```python
from build123d import *

# Parameters (mm, degrees)
SKETCH1_R           = 3.3274
BOSS_EXTRUDE1_DEPTH = 19.05


with BuildPart() as part:
    # Sketch1 → Boss-Extrude1 (new body, symmetric)
    with BuildSketch(Plane.XY):
        with BuildLine():
            Line((-4.064, 16.539617552), (-4.064, 17.496382454))
            ThreePointArc((-4.064, 17.496382454), (-4.519044044, 18.594955958), (-5.617617547, 19.050000004))
            Line((-5.617617547, 19.050000004), (-15.84748704, 19.050000004))
            ThreePointArc((-15.84748704, 19.050000004), (-18.12017629, 18.120192086), (-19.050000001, 15.847509297))
            Line((-19.050000001, 15.847509297), (-19.050000001, 5.617617549))
            ThreePointArc((-19.050000001, 5.617617549), (-18.594955957, 4.519044045), (-17.496382454, 4.064))
            Line((-17.496382454, 4.064), (-16.539617549, 4.064))
            ThreePointArc((-16.539617549, 4.064), (-15.441044044, 4.519044045), (-14.986, 5.617617549))
            Line((-14.986, 5.617617549), (-14.986, 9.385342517))
            ThreePointArc((-14.986, 9.385342517), (-14.721898184, 10.022940701), (-14.0843, 10.287042517))
            Line((-14.0843, 10.287042517), (-13.516042086, 10.287042517))
            ThreePointArc((-13.516042086, 10.287042517), (-13.170975923, 10.218404479), (-12.878443117, 10.022939917))
            Line((-12.878443117, 10.022939917), (-8.14758008, 5.292065242))
            ThreePointArc((-8.14758008, 5.292065242), (-7.117955877, 3.751120652), (-6.756399998, 1.933453582))
            Line((-6.756399998, 1.933453582), (-6.756399998, -1.933453584))
            ThreePointArc((-6.756399998, -1.933453584), (-7.117955877, -3.751120652), (-8.147580078, -5.292065242))
            Line((-8.147580078, -5.292065242), (-12.878443116, -10.022939917))
            ThreePointArc((-12.878443116, -10.022939917), (-13.170975922, -10.21840448), (-13.516042086, -10.287042518))
            Line((-13.516042086, -10.287042518), (-14.0843, -10.287042518))
            ThreePointArc((-14.0843, -10.287042518), (-14.721898185, -10.022940703), (-14.986, -9.385342518))
            Line((-14.986, -9.385342518), (-14.986, -5.617617549))
            ThreePointArc((-14.986, -5.617617549), (-15.441044044, -4.519044046), (-16.539617547, -4.064))
            Line((-16.539617547, -4.064), (-17.496382452, -4.064))
            ThreePointArc((-17.496382452, -4.064), (-18.594955956, -4.519044044), (-19.050000001, -5.617617547))
            Line((-19.050000001, -5.617617547), (-19.050000001, -15.84751072))
            ThreePointArc((-19.050000001, -15.84751072), (-18.120175718, -18.120192644), (-15.84748687, -19.050000001))
            Line((-15.84748687, -19.050000001), (-5.617617549, -19.050000001))
            ThreePointArc((-5.617617549, -19.050000001), (-4.519044046, -18.594955957), (-4.064, -17.496382454))
            Line((-4.064, -17.496382454), (-4.064, -16.539617549))
            ThreePointArc((-4.064, -16.539617549), (-4.519044045, -15.441044044), (-5.617617549, -14.985999999))
            Line((-5.617617549, -14.985999999), (-9.3853, -14.985999999))
            ThreePointArc((-9.3853, -14.985999999), (-10.022898185, -14.721898184), (-10.287, -14.084299999))
            Line((-10.287, -14.084299999), (-10.287, -13.552357131))
            ThreePointArc((-10.287, -13.552357131), (-10.218362387, -13.207291993), (-10.022898969, -12.914759731))
            Line((-10.022898969, -12.914759731), (-5.252158104, -8.14400713))
            ThreePointArc((-5.252158104, -8.14400713), (-3.715177371, -7.117027388), (-1.902183976, -6.7564))
            Line((-1.902183976, -6.7564), (1.902183976, -6.7564))
            ThreePointArc((1.902183976, -6.7564), (3.715177372, -7.117027388), (5.252158106, -8.144007132))
            Line((5.252158106, -8.144007132), (10.022898969, -12.91475973))
            ThreePointArc((10.022898969, -12.91475973), (10.218362387, -13.207291993), (10.287000001, -13.552357132))
            Line((10.287000001, -13.552357132), (10.287000001, -14.0843))
            ThreePointArc((10.287000001, -14.0843), (10.022898185, -14.721898184), (9.385300001, -14.986))
            Line((9.385300001, -14.986), (5.617617549, -14.986))
            ThreePointArc((5.617617549, -14.986), (4.519044045, -15.441044044), (4.064, -16.539617547))
            Line((4.064, -16.539617547), (4.064, -17.496382452))
            ThreePointArc((4.064, -17.496382452), (4.519044043, -18.594955955), (5.617617546, -19.050000001))
            Line((5.617617546, -19.050000001), (15.847486867, -19.050000001))
            ThreePointArc((15.847486867, -19.050000001), (18.120175716, -18.120192646), (19.05, -15.847510723))
            Line((19.05, -15.847510723), (19.05, -5.617617549))
            ThreePointArc((19.05, -5.617617549), (18.594955955, -4.519044045), (17.496382451, -4.064))
            Line((17.496382451, -4.064), (16.539617548, -4.064))
            ThreePointArc((16.539617548, -4.064), (15.441044044, -4.519044045), (14.985999999, -5.617617549))
            Line((14.985999999, -5.617617549), (14.985999999, -9.385342517))
            ThreePointArc((14.985999999, -9.385342517), (14.721898184, -10.022940701), (14.084299999, -10.287042517))
            Line((14.084299999, -10.287042517), (13.516042085, -10.287042517))
            ThreePointArc((13.516042085, -10.287042517), (13.170975922, -10.218404479), (12.878443117, -10.022939917))
            Line((12.878443117, -10.022939917), (8.147580079, -5.292065242))
            ThreePointArc((8.147580079, -5.292065242), (7.117955877, -3.751120652), (6.756399998, -1.933453583))
            Line((6.756399998, -1.933453583), (6.756399998, 1.933453583))
            ThreePointArc((6.756399998, 1.933453583), (7.117955877, 3.751120652), (8.147580078, 5.292065242))
            Line((8.147580078, 5.292065242), (12.878443116, 10.022939916))
            ThreePointArc((12.878443116, 10.022939916), (13.170975922, 10.218404477), (13.516042084, 10.287042515))
            Line((13.516042084, 10.287042515), (14.084299998, 10.287042515))
            ThreePointArc((14.084299998, 10.287042515), (14.721898183, 10.0229407), (14.985999998, 9.385342515))
            Line((14.985999998, 9.385342515), (14.985999998, 5.617617546))
            ThreePointArc((14.985999998, 5.617617546), (15.441044043, 4.519044042), (16.539617547, 4.063999997))
            Line((16.539617547, 4.063999997), (17.49638245, 4.063999997))
            ThreePointArc((17.49638245, 4.063999997), (18.594955956, 4.519044042), (19.05, 5.617617548))
            Line((19.05, 5.617617548), (19.05, 15.8475093))
            ThreePointArc((19.05, 15.8475093), (18.120176289, 18.120192086), (15.847487041, 19.050000004))
            Line((15.847487041, 19.050000004), (5.617617548, 19.050000004))
            ThreePointArc((5.617617548, 19.050000004), (4.519044044, 18.594955959), (4.063999999, 17.496382454))
            Line((4.063999999, 17.496382454), (4.063999999, 16.539617552))
            ThreePointArc((4.063999999, 16.539617552), (4.519044044, 15.441044047), (5.617617548, 14.986000002))
            Line((5.617617548, 14.986000002), (9.385299999, 14.986000002))
            ThreePointArc((9.385299999, 14.986000002), (10.022898183, 14.721898187), (10.286999999, 14.084300002))
            Line((10.286999999, 14.084300002), (10.286999999, 13.552357134))
            ThreePointArc((10.286999999, 13.552357134), (10.218362386, 13.207291996), (10.022898968, 12.914759734))
            Line((10.022898968, 12.914759734), (5.252158103, 8.144007133))
            ThreePointArc((5.252158103, 8.144007133), (3.71517737, 7.117027391), (1.902183975, 6.756400003))
            Line((1.902183975, 6.756400003), (-1.902183977, 6.756400003))
            ThreePointArc((-1.902183977, 6.756400003), (-3.715177373, 7.117027391), (-5.252158106, 8.144007134))
            Line((-5.252158106, 8.144007134), (-10.022898969, 12.914759733))
            ThreePointArc((-10.022898969, 12.914759733), (-10.218362387, 13.207291995), (-10.287000001, 13.552357134))
            Line((-10.287000001, 13.552357134), (-10.287000001, 14.084300002))
            ThreePointArc((-10.287000001, 14.084300002), (-10.022898186, 14.721898187), (-9.385300001, 14.986000002))
            Line((-9.385300001, 14.986000002), (-5.617617549, 14.986000002))
            ThreePointArc((-5.617617549, 14.986000002), (-4.519044044, 15.441044047), (-4.064, 16.539617552))
        make_face()
        Circle(SKETCH1_R, mode=Mode.SUBTRACT)
    extrude(amount=BOSS_EXTRUDE1_DEPTH, both=True)


solid = part.part
```
For this review, take the finished solid that the model builds, in its own axes (mm). A direction names the side the tool comes from. Give positions to 0.01 mm unless a question says otherwise; leave off trailing zeros. Order: outer loops, then holes, each group sorted by start corner. A loop starts at its lowest first (then second) coordinate and runs counter-clockwise, first axis right, second up.
1) Take a section at A-A (x = 0). Give the boundary of the cut face in (y, z), then the cut area to 3 significant figures.
2) Insertion check: pin 1 (6 mm diameter, centred on x = -8, y = -12.5, fed in from -Z); pin 2 (0.5 mm diameter, centred on y = 17, z = 3, fed in from -X); pin 3 (1.1 mm diameter, centred on x = -17, z = 0.5, fed in from -Y); pin 4 (0.5 mm diameter, centred on x = -17, z = -2, fed in from +Y). Each pin has a flat end and moves straight along its axis. Give the tip position at first contact, or say it passes through.
3) The part is to be moulded in two halves that separate along X. For faces 3 (the face through (-14.986, 7, 0)), 4 (the face through (18.583, 4.507, 0.267)), 5 (the face through (-5, 0, 19.05)), 6 (the face through (-18.583, -4.507, 0.267)), say which applies: released by +X, released by -X, zero draft, split by the parting line, or undercut.
4) Wall thickness on line 1 (Y direction, x = -6.5, z = -6); line 2 (Y direction, x = 0, z = -7); line 3 (Y direction, x = -9, z = 8): over which ranges is each line inside the solid? List them lowest first.
5) For faces 1 (the face through (-4.51, -15.45, 0.27)), 2 (the face through (11, 19.05, 0)), list the 3-axis set-ups (+Z, -Z, +X, -X, +Y, -Y) from which the entire face can be reached by the end or side of a thin tool; tool diameter is ignored.
6) Take a section at C-C (y = -7.5). Give the boundary of the cut face in (x, z).
Derived:
1. outline: (-6.76, -19.05) - (-3.33, -19.05) - (-3.33, 19.05) - (-6.76, 19.05) - close; (3.33, -19.05) - (6.76, -19.05) - (6.76, 19.05) - (3.33, 19.05) - close
1. area: 261 mm2
2. pin 1: stops at z = -19.05
2. pin 2: stops at x = -18.93
2. pin 3: stops at y = -19
2. pin 4: stops at y = 18.93
3. face 3: undercut
3. face 4: released by +X
3. face 5: zero draft
3. face 6: released by -X
4. line 1: y = -19.05 to -14.99, -9.39 to 9.39, 14.99 to 19.05
4. line 2: y = -6.76 to -3.33, 3.33 to 6.76
4. line 3: y = -19.05 to -14.99, -11.89 to -6.14, 6.14 to 11.89, 14.99 to 19.05
5. face 1: +Z, -Z
5. face 2: +Z, -Z, +X, -X, +Y
6. outline: (-19.05, -19.05) - (-14.99, -19.05) - (-14.99, 19.05) - (-19.05, 19.05) - close; (-10.36, -19.05) - (-4.45, -19.05) - (-4.45, 19.05) - (-10.36, 19.05) - close; (4.45, -19.05) - (10.36, -19.05) - (10.36, 19.05) - (4.45, 19.05) - close; (14.99, -19.05) - (19.05, -19.05) - (19.05, 19.05) - (14.99, 19.05) - close
